from build123d import *

# Parameters (mm, degrees)
BASE_EXTRUDE_DEPTH = 15
HOLE1_OUTLINE_R    = 5
HOLE1_DEPTH        = 15
HOLE2_OUTLINE_R    = 5
HOLE2_DEPTH        = 15
FILLET1_R          = 15
FILLET2_R          = 5
FILLET3_R          = 2


# Read off the part's stored shape, not the designer's step: Hole1, Hole2
with BuildPart() as part:
    # Sketch1 → Base-Extrude (new body)
    with BuildSketch(Plane.XY):
        with BuildLine():
            Line((-8.009157876, 8.252477817), (18, 33.494769435))
            Line((18, 33.494769435), (54, 33.494769435))
            Line((54, 33.494769435), (80.009157876, 8.252477817))
            ThreePointArc((80.009157876, 8.252477817), (80.252477817, -8.009157876), (63.990842124, -8.252477817))
            Line((63.990842124, -8.252477817), (47.25, 7.994769435))
            Line((47.25, 7.994769435), (24.75, 7.994769435))
            Line((24.75, 7.994769435), (8.009157876, -8.252477817))
            ThreePointArc((8.009157876, -8.252477817), (-8.252477817, -8.009157876), (-8.009157876, 8.252477817))
        make_face()
    extrude(amount=BASE_EXTRUDE_DEPTH)

    # Hole1 outline → Hole1 (cut)
    with BuildSketch(Plane.XY):
        Circle(HOLE1_OUTLINE_R)
    extrude(amount=HOLE1_DEPTH, mode=Mode.SUBTRACT)

    # Hole2 outline → Hole2 (cut)
    with BuildSketch(Plane.XY):
        with Locations((72, 0)):
            Circle(HOLE2_OUTLINE_R)
    extrude(amount=HOLE2_DEPTH, mode=Mode.SUBTRACT)

    # Fillet1
    fillet1_edges = [part.edges().sort_by_distance(p)[0] for p in [
        (18, 33.494769435, 7.5),
        (54, 33.494769435, 7.5),
    ]]
    fillet(fillet1_edges, radius=FILLET1_R)

    # Fillet2
    fillet2_edges = [part.edges().sort_by_distance(p)[0] for p in [
        (47.25, 7.994769435, 7.5),
        (24.75, 7.994769435, 7.5),
    ]]
    fillet(fillet2_edges, radius=FILLET2_R)

    # Fillet3
    fillet3_edges = [part.edges().sort_by_distance(p)[0] for p in [
        (15.652147936, -0.834837274, 0),
        (-8.252477817, -8.009157876, 0),
        (80.252477817, -8.009157876, 15),
        (2.813128058, 18.755674377, 15),
        (36, 33.494769435, 0),
        (36, 33.494769435, 15),
        (69.186871942, 18.755674377, 0),
        (18.445720917, 32.395516223, 0),
        (53.554279083, 32.395516223, 0),
        (69.186871942, 18.755674377, 15),
        (18.445720917, 32.395516223, 15),
        (53.554279083, 32.395516223, 15),
        (-8.252477817, -8.009157876, 15),
        (36, 7.994769435, 0),
        (36, 7.994769435, 15),
        (56.347852064, -0.834837274, 0),
        (56.347852064, -0.834837274, 15),
        (24.898573639, 7.628351698, 0),
        (24.898573639, 7.628351698, 15),
        (47.101426361, 7.628351698, 0),
        (47.101426361, 7.628351698, 15),
        (15.652147936, -0.834837274, 15),
        (2.813128058, 18.755674377, 0),
        (80.252477817, -8.009157876, 0),
    ]]
    fillet(fillet3_edges, radius=FILLET3_R)


solid = part.part
The model under review builds one solid part; all positions refer to its coordinate system, in mm. A direction names the side the tool comes from. Give positions to 0.01 mm unless a question says otherwise; leave off trailing zeros. Order: outer loops, then holes, each group sorted by start corner. A loop starts at its lowest first (then second) coordinate and runs counter-clockwise, first axis right, second up. Notation, with made-up numbers: (-38, 10) -> (18, 10) arc R6 cw to (18, 19) -> close; hole circle Ø5 at (0, -2.75). An arc over 180 degrees is marked (long way). Write item = value, one per line. Start each with the question number.
(1) Take a section at D-D (z = 14). Write out the cut boundary in (x, y), plus the area to 3 significant figures.
(2) For L1, parallel to X at y = 2, z = 7.25; L2, parallel to X at y = -1, z = 9; L3, parallel to Y at x = 69.5, z = 14.25, list the stretches that pass through material, from the lowest coordinate up. Write a range as from..to.
(3) Take a section at A-A (z = 8.5). Write out the cut boundary in (x, y), plus the area to 3 significant figures.
(4) Draft analysis for pull direction X (two halves, no side actions). For faces 1 (the cylindrical face through (80.427, -7.826, 7.423)), 2 (the flat face through (37, 11, 0)), 3 (the flat face through (2.662, 18.609, 7.423)), state which applies: +X half, -X half, draft (parallel to the pull), parting line (faces both ways), or undercut.
(5) Take a section at C-C (y = 0). State how many separate pieces and enclosed holes the cut face has, plus the area to 3 significant figures.
(6) For pin 1 Ø12 at (x, y) = (70.5, 3.5) entering from +Z; pin 2 Ø5 at (x, z) = (68, 3) entering from +Y; pin 3 Ø1 at (y, z) = (9.5, 7.5) entering from +X; pin 4 Ø4 at (y, z) = (24.5, 7) entering from -X, all flat-tipped, find the tip position at first contact; note any pin that passes through.
(7) Tool access review of faces 4 (the cylindrical face through (76.619, -1.915, 7.395)), 5 (the cylindrical face through (15.148, -0.529, 14.399)), 6 (the flat face through (36, 7.995, 7)), 7 (the cylindrical face through (56.66, -0.3, 0.57)), 8 (the cylindrical face through (3.38, 18.47, 0.57)): name each direction out of +Z, -Z, +X, -X, +Y, -Y from which nothing blocks a thin tool from reaching the whole face with its end or side.
(8) Take a section at B-B (x = 30). Write out the cut boundary in (y, z).
Returned:
q1.outline = (-7.82, 8.06) arc R11.23 ccw to (7.82, -8.06) -> (23.11, 6.78) arc R5.27 cw to (26.78, 8.26) -> (45.22, 8.26) arc R5.27 cw to (48.89, 6.78) -> (64.18, -8.06) arc R11.23 ccw to (79.82, 8.06) -> (58.18, 29.07) arc R14.73 ccw to (47.92, 33.23) -> (24.08, 33.23) arc R14.73 ccw to (13.82, 29.07) -> close; hole circle Ø10 at (0, 0); hole circle Ø10 at (72, 0)
q1.area = 2,300 mm²
q2.L1 = -11.32..-4.58, 4.58..18.57, 53.43..67.42, 76.58..83.32
q2.L2 = -11.46..-4.9, 4.9..15.48, 56.52..67.1, 76.9..83.46
q2.L3 = -10.78..-4.33, 4.33..17.84
q3.outline = (-8.01, 8.25) arc R11.5 ccw to (8.01, -8.25) -> (23.3, 6.58) arc R5 cw to (26.78, 7.99) -> (45.22, 7.99) arc R5 cw to (48.7, 6.58) -> (63.99, -8.25) arc R11.5 ccw to (80.01, 8.25) -> (58.36, 29.26) arc R15 ccw to (47.92, 33.49) -> (24.08, 33.49) arc R15 ccw to (13.64, 29.26) -> close; hole circle Ø10 at (0, 0); hole circle Ø10 at (72, 0)
q3.area = 2,370 mm²
q4.face_1 = undercut
q4.face_2 = draft
q4.face_3 = -X half
q5.separate_pieces = 4
q5.enclosed_holes = 0
q5.area = 532 mm²
q6.pin_1 = 15
q6.pin_2 = 22.33
q6.pin_3 = 79.24
q6.pin_4 = 6.67
q7.face_4 = +Z, -Z
q7.face_5 = +Z, -Y
q7.face_6 = +Z, -Z, -Y
q7.face_7 = -Z, -Y
q7.face_8 = -Z, -X, +Y
q8.outline = (7.99, 2) arc R2 ccw to (9.99, 0) -> (31.49, 0) arc R2 ccw to (33.49, 2) -> (33.49, 13) arc R2 ccw to (31.49, 15) -> (9.99, 15) arc R2 ccw to (7.99, 13) -> close
